```python
from build123d import *

# Parameters (mm, degrees)
BOSS_EXTRUDE1_DEPTH             = 6.35
F_1_4_0_25_DIAMETER_HOLE1_D     = 6.35
F_1_4_0_25_DIAMETER_HOLE1_DEPTH = 16.51
F_1_4_0_25_DIAMETER_HOLE1_TIP   = 1.907732465
F_8_CLEARANCE_HOLE1_D           = 4.4958
F_8_CLEARANCE_HOLE1_DEPTH       = 16.51
F_8_CLEARANCE_HOLE1_TIP         = 1.350674586
SKETCH7_R                       = 4.7625
CUT_EXTRUDE1_DEPTH              = 7.35
CUT_EXTRUDE2_DEPTH              = 7.35
SKETCH9_R                       = 8.89
CUT_EXTRUDE3_DEPTH              = 7.35


with BuildPart() as part:
    # Sketch1 → Boss-Extrude1 (new body)
    with BuildSketch(Plane(origin=(0, 0, 0), x_dir=(1, 0, 0), z_dir=(0, 1, 0))):
        with BuildLine():
            Line((-52.3875, -42.8625), (-52.3875, 0))
            ThreePointArc((-52.3875, 0), (-51.5575956, 3.888564967), (-49.2125, 7.099515829))
            Line((-49.2125, 7.099515829), (-25.4, 28.398063314))
            ThreePointArc((-25.4, 28.398063314), (15.554259867, 34.780382402), (38.1, 0))
            Line((38.1, 0), (38.1, -42.8625))
            Line((38.1, -42.8625), (-52.3875, -42.8625))
        make_face()
    extrude(amount=BOSS_EXTRUDE1_DEPTH)

    # 1/4 (0.25) Diameter Hole1
    with Locations(Plane(origin=(0, 6.35, 0), x_dir=(1, 0, 0), z_dir=(0, 1, 0))):
        with Locations((-42.8625, 0)):
            Hole(F_1_4_0_25_DIAMETER_HOLE1_D / 2, depth=F_1_4_0_25_DIAMETER_HOLE1_DEPTH)
            with Locations((0, 0, -(F_1_4_0_25_DIAMETER_HOLE1_DEPTH + F_1_4_0_25_DIAMETER_HOLE1_TIP / 2))):  # 118° drill point
                Cone(0, F_1_4_0_25_DIAMETER_HOLE1_D / 2, F_1_4_0_25_DIAMETER_HOLE1_TIP, mode=Mode.SUBTRACT)

    # #8 Clearance Hole1
    with Locations(Plane(origin=(0, 6.35, 0), x_dir=(1, 0, 0), z_dir=(0, 1, 0))):
        with Locations((-46.0375, -39.6875), (-20.6375, -39.6875)):
            Hole(F_8_CLEARANCE_HOLE1_D / 2, depth=F_8_CLEARANCE_HOLE1_DEPTH)
            with Locations((0, 0, -(F_8_CLEARANCE_HOLE1_DEPTH + F_8_CLEARANCE_HOLE1_TIP / 2))):  # 118° drill point
                Cone(0, F_8_CLEARANCE_HOLE1_D / 2, F_8_CLEARANCE_HOLE1_TIP, mode=Mode.SUBTRACT)

    # Sketch7 → Cut-Extrude1 (cut, through all)
    with BuildSketch(Plane(origin=(0, 6.35, 0), x_dir=(1, 0, 0), z_dir=(0, 1, 0))):
        Circle(SKETCH7_R)
    extrude(amount=-CUT_EXTRUDE1_DEPTH, mode=Mode.SUBTRACT)

    # Sketch8 → Cut-Extrude2 (cut, through all)
    with BuildSketch(Plane(origin=(0, 6.35, 0), x_dir=(1, 0, 0), z_dir=(0, 1, 0))):
        with BuildLine():
            Line((-14.2875, -42.8625), (9.267264347, -36.955754782))
            ThreePointArc((9.267264347, -36.955754782), (30.039080975, -23.436373742), (38.1, 0))
            Line((38.1, 0), (38.1, -42.8625))
            Line((38.1, -42.8625), (-14.2875, -42.8625))
        make_face()
    extrude(amount=-CUT_EXTRUDE2_DEPTH, mode=Mode.SUBTRACT)

    # Sketch9 → Cut-Extrude3 (cut, through all)
    with BuildSketch(Plane(origin=(0, 6.35, 0), x_dir=(1, 0, 0), z_dir=(0, 1, 0))):
        with Locations((-22.225, 0)):
            Circle(SKETCH9_R)
        with Locations((-11.1125, 19.247414599)):
            Circle(SKETCH9_R)
        with Locations((11.1125, 19.247414599)):
            Circle(SKETCH9_R)
        with Locations((22.225, 0)):
            Circle(SKETCH9_R)
        with Locations((11.1125, -19.247414599)):
            Circle(SKETCH9_R)
        with Locations((-11.1125, -19.247414599)):
            Circle(SKETCH9_R)
        with BuildLine():
            Line((-42.8625, -12.934062773), (-42.8625, -30.1625))
            ThreePointArc((-42.8625, -30.1625), (-41.93256403, -32.40756403), (-39.6875, -33.3375))
            Line((-39.6875, -33.3375), (-29.740657129, -33.3375))
            ThreePointArc((-29.740657129, -33.3375), (-26.991026472, -31.75), (-26.991026472, -28.575))
            Line((-26.991026472, -28.575), (-36.937869343, -11.346562773))
            ThreePointArc((-36.937869343, -11.346562773), (-40.509250468, -9.867248274), (-42.8625, -12.934062773))
        make_face()
    extrude(amount=-CUT_EXTRUDE3_DEPTH, mode=Mode.SUBTRACT)


solid = part.part
```
Design review of the part built by this model. Coordinates are the model's own, in mm. A direction names the side the tool comes from. Give positions to 0.01 mm unless a question says otherwise; leave off trailing zeros. Loops run counter-clockwise (first coordinate to the right, second up) from the corner with the lowest first, then second, coordinate; pieces in that order, holes last. Notation, with made-up numbers: (85.5, 44.5) -> (91.5, 44.5) arc R24 cw to (91.5, 68.5) -> close; hole circle Ø9 at (15.5, 24). An arc over 180 degrees is marked (long way). One line per item, written item: value.
Q1. Machinability: for faces 1 (the cylindrical face through (-40.45, 3.22, 9.85)), 2 (the flat face through (-52.388, 3, 22)), which of the approach directions +Z, -Z, +X, -X, +Y, -Y give a long, thin tool a straight path to every point of the face, cutting with its end or side? Answer none if there is none.
Numbers:
face 1: +Y, -Y
face 2: +Z, -Z, -X, +Y, -Y
Q2. We need section A-A on x = -28. Give the boundary of the cut face in (y, z).
Numbers:
outline: (0, -26.07) -> (6.35, -26.07) -> (6.35, -6.76) -> (0, -6.76) -> close; (0, 6.76) -> (6.35, 6.76) -> (6.35, 26.83) -> (0, 26.83) -> close; (0, 32.82) -> (6.35, 32.82) -> (6.35, 42.86) -> (0, 42.86) -> close
Q3. Draft analysis for pull direction Z (two halves, no side actions). For faces 3 (the cylindrical face through (-51.58, 3.13, -3.84)), 4 (the cylindrical face through (15.215, 3.219, 27.134)), 5 (the flat face through (-7, 0, 2)), state which applies: pulls with the +Z half, pulls with the -Z half, needs draft (parallel to the pull), parting line crosses it, or undercut.
Numbers:
face 3: pulls with the -Z half
face 4: undercut
face 5: needs draft
Q4. For pin 1 Ø3 at (y, z) = (4.5, -16.5) entering from -X; pin 2 Ø20.5 at (x, z) = (11.11, 19.25) entering from +Y; pin 3 Ø1.5 at (x, y) = (-34, 3) entering from -Z; pin 4 Ø2 at (x, y) = (4.5, 3.5) entering from -Z, all flat-tipped, find the tip position at first contact; note any pin that passes through.
Numbers:
pin 1: stops at x = -40.38
pin 2: stops at y = 6.35
pin 3: stops at z = -21.38
pin 4: stops at z = -37.94
Q5. We need section C-C on x = 0. Give the boundary of the cut face in (y, z).
Numbers:
outline: (0, -38.1) -> (6.35, -38.1) -> (6.35, -4.76) -> (0, -4.76) -> close; (0, 4.76) -> (6.35, 4.76) -> (6.35, 39.28) -> (0, 39.28) -> close
Q6. We need section B-B on y = 3.75. Give the number of separate pieces and of enclosed holes in the cut face, and give its area (3 significant figures).
Numbers:
separate pieces: 1
enclosed holes: 11
area: 3,940 mm^2
Q7. For L1, parallel to Z at x = -22.5, y = 2.75; L2, parallel to Z at x = 12, y = 0.5; L3, parallel to X at y = 4.25, z = 6.5, list the stretches that pass through material, from the lowest coordinate up.
Numbers:
L1: z = -30.75 to -8.89, 8.89 to 38.43, 40.95 to 42.86
L2: z = -36.16 to -28.09, -10.4 to 10.4, 28.09 to 36.16
L3: x = -52.39 to -28.29, -16.16 to 16.16, 28.29 to 37.54
